```python
from build123d import *

# Parameters (mm, degrees)
SKETCH1_W           = 54
SKETCH1_H           = 54
SKETCH1_R           = 2.75
BOSS_EXTRUDE1_DEPTH = 5
FILLET1_R           = 8
FILLET2_R           = 0.5
FILLET3_R           = 1
SKETCH2_R           = 4.5
CUT_EXTRUDE2_DEPTH  = 2


with BuildPart() as part:
    # Sketch1 → Boss-Extrude1 (new body)
    with BuildSketch(Plane.XY):
        Rectangle(SKETCH1_W, SKETCH1_H)
        with Locations((-19, 19)):
            Circle(SKETCH1_R, mode=Mode.SUBTRACT)
        with Locations((19, 19)):
            Circle(SKETCH1_R, mode=Mode.SUBTRACT)
        with Locations((19, -19)):
            Circle(SKETCH1_R, mode=Mode.SUBTRACT)
        with Locations((-19, -19)):
            Circle(SKETCH1_R, mode=Mode.SUBTRACT)
    extrude(amount=BOSS_EXTRUDE1_DEPTH)

    # Fillet1
    fillet1_edges = [part.edges().sort_by_distance(p)[0] for p in [
        (-27, 27, 2.5),
        (27, 27, 2.5),
        (27, -27, 2.5),
        (-27, -27, 2.5),
    ]]
    fillet(fillet1_edges, radius=FILLET1_R)

    # Fillet2
    fillet2_edges = [part.edges().sort_by_distance(p)[0] for p in [
        (-21.75, 19, 0),
        (-21.75, 19, 5),
        (16.25, 19, 0),
        (16.25, 19, 5),
        (16.25, -19, 0),
        (16.25, -19, 5),
        (-21.75, -19, 0),
        (-21.75, -19, 5),
    ]]
    fillet(fillet2_edges, radius=FILLET2_R)

    # Fillet3
    fillet3_edges = [part.edges().sort_by_distance(p)[0] for p in [
        (-27, 0, 5),
        (0, 27, 5),
        (0, -27, 5),
        (27, 0, 5),
        (24.656854249, 24.656854249, 5),
        (-24.656854249, -24.656854249, 5),
        (24.656854249, -24.656854249, 5),
        (-24.656854249, 24.656854249, 5),
    ]]
    fillet(fillet3_edges, radius=FILLET3_R)

    # Sketch2 → Cut-Extrude2 (cut)
    with BuildSketch(Plane.XY.offset(5)):
        with Locations((-19, 19)):
            Circle(SKETCH2_R)
        with Locations((19, 19)):
            Circle(SKETCH2_R)
        with Locations((19, -19)):
            Circle(SKETCH2_R)
        with Locations((-19, -19)):
            Circle(SKETCH2_R)
    extrude(amount=-CUT_EXTRUDE2_DEPTH, mode=Mode.SUBTRACT)


solid = part.part
```
For this review, take the finished solid that the model builds, in its own axes (mm). A direction names the side the tool comes from. Give positions to 0.01 mm unless a question says otherwise; leave off trailing zeros. One line per item, written item: value. Start each with the question number.
Q1. Clearance check with flat-ended pins moving along their axes: pin 1 Ø10 at (x, y) = (15, -19) entering from +Z; pin 2 Ø6.5 at (x, y) = (19, -19) entering from +Z; pin 3 Ø3.5 at (x, y) = (-19, 19) entering from +Z. State where each tip first meets the part, or that it passes through.
Q2. Machinability: for faces 4 (the face through (24.594, 24.719, 2.028)), 5 (the face through (-19, -22, 3)), which of the approach directions +Z, -Z, +X, -X, +Y, -Y give a long, thin tool a straight path to every point of the face, cutting with its end or side? Answer none if there is none.
Q3. Draft analysis for pull direction X (two halves, no side actions). For faces 1 (the face through (-24.719, -24.594, 2.028)), 2 (the face through (0, 0, 5)), 3 (the face through (15.68, 22.04, 4.01)), state which applies: released by +X, released by -X, zero draft, split by the parting line, or undercut.
Q4. Add section A-A (x = 18). Count the separate pieces of the cut face and the enclosed holes in it, and give its area (3 significant figures).
Q5. For L1, parallel to Y at x = 19, z = 1.75; L2, parallel to Y at x = -19, z = 4.45, list the stretches that pass through material, from the lowest coordinate up.
Reply:
1. pin 1: z = 5
1. pin 2: z = 3
1. pin 3: through
2. face 4: +Z, -Z, +X, +Y
2. face 5: +Z
3. face 1: released by -X
3. face 2: zero draft
3. face 3: undercut
4. separate pieces: 3
4. enclosed holes: 0
4. area: 204 mm²
5. L1: -27 to -21.75, -16.25 to 16.25, 21.75 to 27
5. L2: -26.89 to -23.5, -14.5 to 14.5, 23.5 to 26.89
